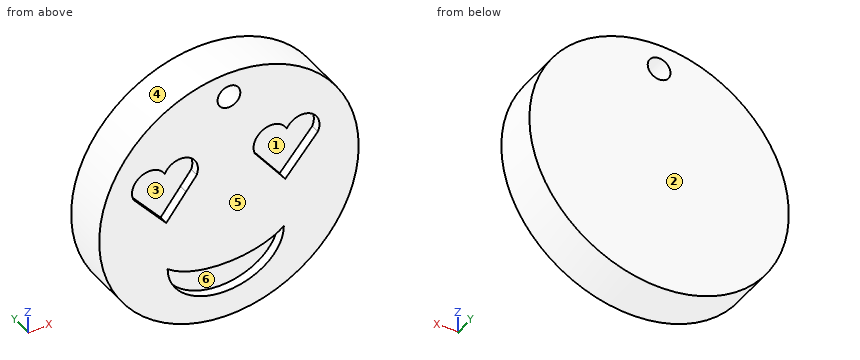
from build123d import *

# Parameters (mm, degrees)
F0_R     = 35.9731805371
F1_DEPTH = 12.7
F3_DEPTH = 2.54
F4_R     = 3.1591269053
F5_DEPTH = 12.7


with BuildPart() as f1:
    # F0 (on Front) → F1 (new body)
    with BuildSketch(Plane.XZ):
        Circle(F0_R)
    extrude(amount=F1_DEPTH)

    # F2 (on face) → F3 (cut)
    with BuildSketch(Plane.XZ.offset(12.7)):
        with BuildLine():
            add(Edge.make_bspline(
                [(-16.9929389652, -15.6046478078), (-8.5501303198, -22.0675654258), (8.323411948, -21.2654638787), (15.2166548375, -15.6046478078)],
                knots=[0, 0, 0, 0, 0.2892568057, 0.2892568057, 0.2892568057, 0.2892568057], degree=3))
            add(Edge.make_bspline(
                [(-16.9929389652, -15.6046478078), (-16.9929389652, -28.5709049037), (-0.8881420638, -28.5709049037), (15.2166548375, -28.5709049037), (15.2166548375, -15.6046478078)],
                knots=[3.1415926536, 3.1415926536, 3.1415926536, 4.7123889804, 4.7123889804, 6.2831853072, 6.2831853072, 6.2831853072], degree=2, weights=[1, 0.7071067812, 1, 0.7071067812, 1]))
        make_face()
        with BuildLine():
            Line((-26.4401481881, 8.735650257), (-20.4888275084, 1.8568773465))
            add(Edge.make_bspline(
                [(-11.8826347663, 5.4031915978), (-15.0818594553, 5.0135593832), (-18.2480697552, 3.9656430572), (-20.2552859644, 2.1019215063), (-20.4888275084, 1.8568773465)],
                knots=[0.7025224358, 0.7025224358, 0.7025224358, 0.7025224358, 0.7815743868, 0.7928961202, 0.7928961202, 0.7928961202, 0.7928961202], degree=3))
            Line((-11.8826347663, 5.4031915978), (-8.9330095374, 9.2211581919))
            ThreePointArc((-8.9330095374, 9.2211581919), (-11.5064602723, 15.4265381827), (-17.8002578016, 13.0776017904))
            ThreePointArc((-17.8002578016, 13.0776017904), (-24.2145633889, 15.0741170918), (-26.4401481881, 8.735650257))
        make_face()
        with BuildLine():
            add(Edge.make_bspline(
                [(-11.8826347663, 5.4031915978), (-15.0818594553, 5.0135593832), (-18.2480697552, 3.9656430572), (-20.2552859644, 2.1019215063), (-20.4888275084, 1.8568773465)],
                knots=[0.7025224358, 0.7025224358, 0.7025224358, 0.7025224358, 0.7815743868, 0.7928961202, 0.7928961202, 0.7928961202, 0.7928961202], degree=3))
            Line((-20.4888275084, 1.8568773465), (-17.3897475746, -1.7251623794))
            Line((-17.3897475746, -1.7251623794), (-11.8826347663, 5.4031915978))
        make_face()
        with BuildLine():
            ThreePointArc((24.6638640604, 8.735650257), (22.4382792612, 15.0741170918), (16.0239736739, 13.0776017904))
            ThreePointArc((16.0239736739, 13.0776017904), (9.7301761446, 15.4265381827), (7.1567254097, 9.2211581919))
            Line((7.1567254097, 9.2211581919), (15.6134634469, -1.7251623794))
            Line((15.6134634469, -1.7251623794), (24.6638640604, 8.735650257))
        make_face()
    extrude(amount=-F3_DEPTH, mode=Mode.SUBTRACT)

    # F4 (on Front) → F5 (cut)
    with BuildSketch(Plane.XZ):
        with Locations((0, 28.9524216205)):
            Circle(F4_R)
    extrude(amount=F5_DEPTH, mode=Mode.SUBTRACT)


solid = f1.part
Geometry: final body of the model. Coordinates: model frame, mm. Face numbers are marked on the shaded views. A direction names the side the tool comes from. Give positions to 0.01 mm unless a question says otherwise; leave off trailing zeros. Write each loop counter-clockwise with the first axis right and the second up, starting at its lowest first coordinate (ties: lowest second). Pieces come first, ordered by that corner, then holes. Notation, with made-up numbers: M 46.5,79.5 L 91.5,79.5 A22 ccw 91.5,86.5 Z; hole C 47,66.5 d9. An arc over 180 degrees is marked long. Answer in a Markdown table with one row per item. Add a question column.
(1) Section B-B on y = -6. Return loops of the section in (x, z), and give its area (3 significant figures).
(2) Section C-C on x = -25. Return loops of the section in (y, z).
(3) Section A-A on z = 3. Return loops of the section in (x, y).
(4) Section D-D on y = -11.25. State how many separate pieces and enclosed holes the cut face has, and give its area (3 significant figures).
(5) Mould query, pull axis Z, two halves, no side actions, for the marked faces 3, 4, 5 and 6. Classes: +Z half, -Z half, draft (parallel to the pull), parting line (faces both ways), or undercut.
(6) Reachability of the marked faces 1 and 2 from +Z, -Z, +X, -X, +Y, -Y: full face, straight path, thin tool, end or side. Return the list, or none.
(7) Ray query, line 1 (Z direction, x = 0, y = -6); line 2 (X direction, y = -12, z = 4.5); line 3 (X direction, y = -12, z = 13.5). Return the intervals inside material, ascending.
(8) First-contact query: pin 1 (1 mm diameter, centred on y = -9, z = 27, fed in from -X); pin 2 (1 mm diameter, centred on x = -21, y = -3.5, fed in from -Z); pin 3 (6 mm diameter, centred on x = 28, y = -3.5, fed in from -Z). Flat tips, straight axial feed; report the tip coordinate or a pass-through.
Result set:
| question | item | result |
|---|---|---|
| 1 | outline | C 0,0 d71.95; hole C 0,28.95 d6.32 |
| 1 | area | 4,030 mm^2 |
| 2 | outline | M -12.7,-25.87 L 0,-25.87 L 0,25.87 L -12.7,25.87 L -12.7,14.58 L -10.16,14.58 L -10.16,7.07 L -12.7,7.07 Z |
| 3 | outline | M -35.85,-12.7 L -21.48,-12.7 L -21.48,-10.16 L -13.74,-10.16 L -13.74,-12.7 L 11.96,-12.7 L 11.96,-10.16 L 19.7,-10.16 L 19.7,-12.7 L 35.85,-12.7 L 35.85,0 L -35.85,0 Z |
| 4 | separate pieces | 1 |
| 4 | enclosed holes | 4 |
| 4 | area | 3,410 mm^2 |
| 5 | face 3 | undercut |
| 5 | face 4 | parting line |
| 5 | face 5 | draft |
| 5 | face 6 | undercut |
| 6 | face 1 | -Y |
| 6 | face 2 | +Z, -Z, +X, -X, +Y |
| 7 | line 1 | z = -35.97 to 25.79, 32.11 to 35.97 |
| 7 | line 2 | x = -35.69 to -22.78, -12.58 to 10.8, 21 to 35.69 |
| 7 | line 3 | x = -33.34 to -26.02, -18.06 to -17.57, -9.3 to 7.52, 15.8 to 16.28, 24.25 to 33.34 |
| 8 | pin 1 | stops at x = -24.33 |
| 8 | pin 2 | stops at z = -29.56 |
| 8 | pin 3 | stops at z = -25.87 |
